Geometry check sheet. Reference: the model listing, model coordinates, mm. Face numbers are marked on the shaded views. A direction names the side the tool comes from. Coordinates: 2 decimals unless noted, no trailing zeros. Order: outer loops, then holes, each group sorted by start corner. A loop starts at its lowest first (then second) coordinate and runs counter-clockwise, first axis right, second up. Notation, with made-up numbers: (85.5, -3) - (113.5, -3) arc R16 ccw to (113.5, 10) - close; hole circle Ø2 at (11, 70.5). An arc over 180 degrees is marked (long way). Return JSON: item names as keys, results as strings. Group by question number.
Item 1: Section check C-C on y = 15. Enter the section's corners in (x, z).
Item 2: Tool access check on the marked faces 4, 5, 6, 7 and 8. Record the directions out of +Z, -Z, +X, -X, +Y, -Y that give a thin tool (end or side, any length) a straight path to the whole face; none if there is none.
Item 3: Section check A-A on y = 9.5. Enter the section's corners in (x, z).
Item 4: Draft check along X on the marked faces 1, 2 and 3. Enter one of: pulls with the +X half, pulls with the -X half, needs draft (parallel to the pull), parting line crosses it, or undercut.
Item 5: Scan lines: probe 1 along X at (y, z) = (6, -5); probe 2 along Y at (x, z) = (-7.25, 0); probe 3 along Y at (x, z) = (2.6, 0). Record each from-to range of solid material in increasing order.
Item 6: Gauge pin test, flat ends, axial feed: pin 1 (8 mm diameter, centred on x = -4, z = -5.5, fed in from +Y); pin 2 (4.5 mm diameter, centred on x = -5, y = 12, fed in from +Z); pin 3 (3 mm diameter, centred on x = -10, z = -10.5, fed in from +Y); pin 4 (6.5 mm diameter, centred on y = 17.5, z = 3, fed in from +X). Record the tip position at first contact, or that the pin passes through.
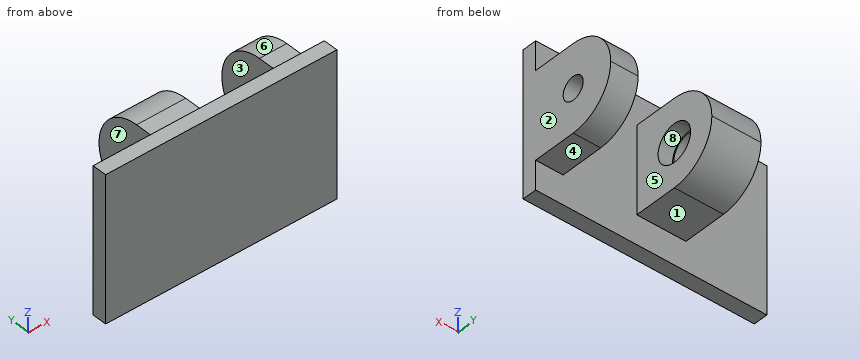
from build123d import *

# Parameters (mm, degrees)
SKETCH1_W           = 80
SKETCH1_H           = 50
BOSS_EXTRUDE1_DEPTH = 5
SKETCH2_W           = 17
SKETCH2_H           = 30
SKETCH2_W_2         = 9.5
BOSS_EXTRUDE2_DEPTH = 30
FILLET1_R           = 15
SKETCH3_R           = 4
CUT_EXTRUDE1_DEPTH  = 30
SKETCH4_R           = 6.5
CUT_EXTRUDE2_DEPTH  = 5
SKETCH5_R           = 6
CUT_EXTRUDE3_DEPTH  = 14


with BuildPart() as part:
    # Sketch1 → Boss-Extrude1 (new body)
    with BuildSketch(Plane(origin=(0, 0, 0), x_dir=(1, 0, 0), z_dir=(0, 1, 0))):
        Rectangle(SKETCH1_W, SKETCH1_H)
    extrude(amount=BOSS_EXTRUDE1_DEPTH)

    # Sketch2 → Boss-Extrude2 (add)
    with BuildSketch(Plane(origin=(0, 5, 0), x_dir=(1, 0, 0), z_dir=(0, 1, 0))):
        with Locations((-3.5, 0)):
            Rectangle(SKETCH2_W, SKETCH2_H)
        with Locations((35.25, 0)):
            Rectangle(SKETCH2_W_2, SKETCH2_H)
    extrude(amount=BOSS_EXTRUDE2_DEPTH)

    # Fillet1
    fillet1_edges = [part.edges().sort_by_distance(p)[0] for p in [
        (-3.5, 35, -15),
        (-3.5, 35, 15),
        (35.25, 35, -15),
        (35.25, 35, 15),
    ]]
    fillet(fillet1_edges, radius=FILLET1_R - 0.0001)  # a hair under: the kernel refuses the full size

    # Sketch3 → Cut-Extrude1 (cut)
    with BuildSketch(Plane.ZY.offset(-30.5)):
        with Locations((0, 20)):
            Circle(SKETCH3_R)
    extrude(amount=-CUT_EXTRUDE1_DEPTH, mode=Mode.SUBTRACT)

    # Sketch4 → Cut-Extrude2 (cut)
    with BuildSketch(Plane(origin=(5, 0, 0), x_dir=(0, 0, -1), z_dir=(1, 0, 0))):
        with Locations((0, 20)):
            Circle(SKETCH4_R)
    extrude(amount=-CUT_EXTRUDE2_DEPTH, mode=Mode.SUBTRACT)

    # Sketch5 → Cut-Extrude3 (cut)
    with BuildSketch(Plane.ZY.offset(12)):
        with Locations((0, 20)):
            Circle(SKETCH5_R)
    extrude(amount=-CUT_EXTRUDE3_DEPTH, mode=Mode.SUBTRACT)


solid = part.part
Computed:
{
 "1": {"outline": "(-12, -15) - (5, -15) - (5, -4.15) - (0, -4.15) - (0, -3.32) - (-12, -3.32) - close; (-12, 3.32) - (0, 3.32) - (0, 4.15) - (5, 4.15) - (5, 15) - (-12, 15) - close; (30.5, -15) - (40, -15) - (40, 15) - (30.5, 15) - close"},
 "2": {"face 4": "-Z, +X, -X, +Y", "face 5": "+Z, -Z, +Y", "face 6": "+Z, +X, -X, +Y", "face 7": "+Z, -Z, -X, +Y", "face 8": "none"},
 "3": {"outline": "(-12, -15) - (5, -15) - (5, 15) - (-12, 15) - close; (30.5, -15) - (40, -15) - (40, 15) - (30.5, 15) - close"},
 "4": {"face 1": "needs draft", "face 2": "pulls with the +X half", "face 3": "undercut"},
 "5": {"probe 1": "x = -12 to 5, 30.5 to 40", "probe 2": "y = 0 to 14, 26 to 35", "probe 3": "y = 0 to 13.5, 26.5 to 35"},
 "6": {"pin 1": "stops at y = 34.92", "pin 2": "stops at z = 15", "pin 3": "stops at y = 32", "pin 4": "stops at x = 40"}
}
